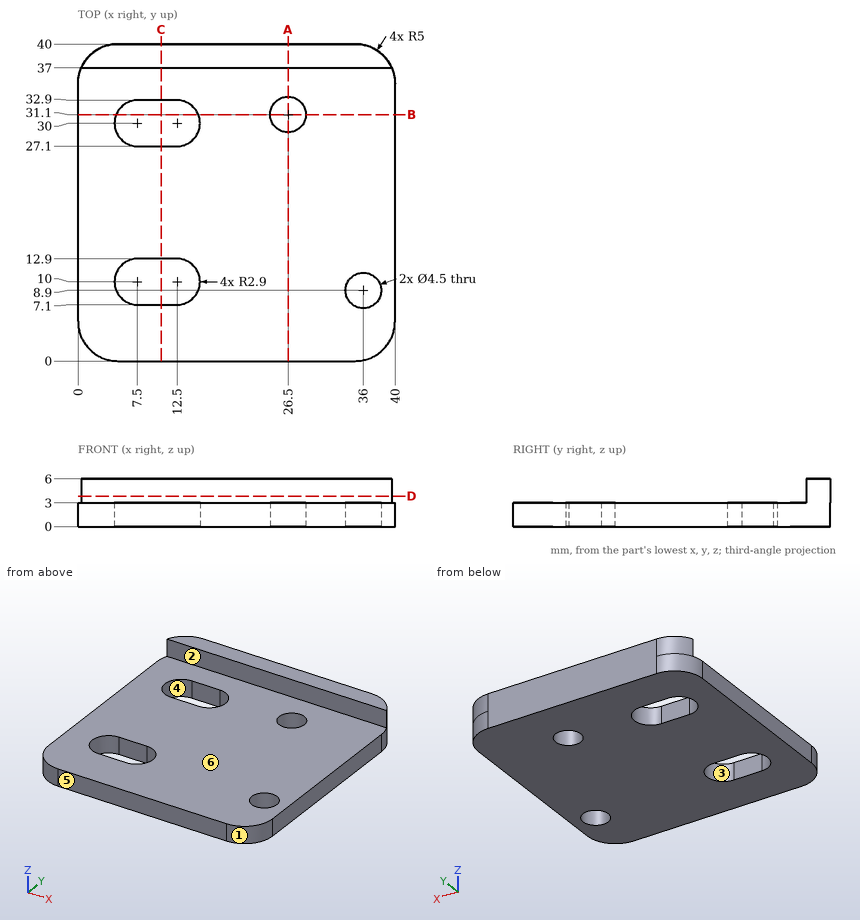
Study the drawing (mm; zero at the part's minimum x, y, z) and answer. A direction names the side the tool comes from. Give positions to 0.01 mm unless a question says otherwise; leave off trailing zeros. Write each loop counter-clockwise with the first axis right and the second up, starting at its lowest first coordinate (ties: lowest second). Pieces come first, ordered by that corner, then holes. Notation, with made-up numbers: (-35, 42) -> (13, 42) arc R25 ccw to (13, 81) -> close; hole circle Ø2 at (47.25, 1.25). An arc over 180 degrees is marked (long way). Write item = value, one per line.
Q1. Flat-ended cylindrical pins translate along their axes: pin 1 Ø2 at (y, z) = (27, 5) entering from +X; pin 2 Ø10 at (x, y) = (12.5, 31) entering from +Z. Find the tip coordinate at first contact, or state that the pin passes through.
Computed values:
pin_1 = through
pin_2 = 3
Q2. Section D-D on z = 3.85 is taken. Determine the outline of the cut face in (x, y).
Computed values:
outline = (0.42, 37) -> (39.58, 37) arc R5 ccw to (35, 40) -> (5, 40) arc R5 ccw to start
Q3. Section C-C on x = 10.5 is taken. Determine the outline of the cut face in (y, z).
Computed values:
outline = (0, 0) -> (7.1, 0) -> (7.1, 3) -> (0, 3) -> close; (12.9, 0) -> (27.1, 0) -> (27.1, 3) -> (12.9, 3) -> close; (32.9, 0) -> (40, 0) -> (40, 6) -> (37, 6) -> (37, 3) -> (32.9, 3) -> close
Q4. Section A-A on x = 26.5 is taken. Determine the outline of the cut face in (y, z).
Computed values:
outline = (0, 0) -> (28.85, 0) -> (28.85, 3) -> (0, 3) -> close; (33.35, 0) -> (40, 0) -> (40, 6) -> (37, 6) -> (37, 3) -> (33.35, 3) -> close
Q5. Section B-B on y = 31.1 is taken. Determine the outline of the cut face in (x, z).
Computed values:
outline = (0, 0) -> (4.82, 0) -> (4.82, 3) -> (0, 3) -> close; (15.18, 0) -> (24.25, 0) -> (24.25, 3) -> (15.18, 3) -> close; (28.75, 0) -> (40, 0) -> (40, 3) -> (28.75, 3) -> close
Q6. Consider line 1 along Y through (x, z) = (14, 2.2); line 2 along Z through (x, y) = (15, 3.5); line 3 along Y through (x, z) = (5.5, 4). Determine where each line is inside the solid, lowest interval first.
Computed values:
line_1 = 0 to 7.52, 12.48 to 27.52, 32.48 to 40
line_2 = 0 to 3
line_3 = 37 to 40
Q7. For a pull along Y with two mould halves and no side action, classify the marked faces 4, 5 and 6 as pulls with the +Y half, pulls with the -Y half, needs draft (parallel to the pull), parting line crosses it, or undercut.
Computed values:
face_4 = undercut
face_5 = pulls with the -Y half
face_6 = needs draft
Q8. A tool of negligible diameter and unlimited length cuts with its end or side. For the marked faces 1, 2 and 3, from which of +Z, -Z, +X, -X, +Y, -Y can it reach the whole face along a straight path? Write none if from no direction.
Computed values:
face_1 = +Z, -Z, +X, -Y
face_2 = +Z, +X, -X, -Y
face_3 = +Z, -Z
